Work out the finished part from the listing and answer in its coordinate system (mm). Face numbers are marked on the shaded views. A direction names the side the tool comes from. Round coordinates to 2 decimals unless told otherwise and drop trailing zeros. Write each loop counter-clockwise with the first axis right and the second up, starting at its lowest first coordinate (ties: lowest second). Pieces come first, ordered by that corner, then holes. Notation, with made-up numbers: (-22.5, 42) -> (-16.5, 42) arc R9 ccw to (-16.5, 54) -> close; hole circle Ø9 at (-3.5, 68). An arc over 180 degrees is marked (long way). One line per item, written item: value.
Solid Edge part; units mm, degrees
sketch "Sketch1" plane through (0, 0, 0) normal (1, 0, 0) x (0, 1, 0)
  line L0 (0, -1.4097) -> (0, 1.4097)
  arc A0 (0, 1.4097) -> (5.25, -1.4097) centre (0.36, -4.2176) cw
  line L1 (0, -1.4097) -> (5.25, -1.4097)
revolve "RevolvedProtrusion1" add sketch "Sketch1" angle 360 about axis through (0, 0, -14.7796) along (0, 0, 1)
sketch "Sketch2" plane through (0, 0, -1.4097) normal (0, 0, -1) x (0, 1, 0)
  circle A0 centre (0, 0) radius 3
extrude "Protrusion1" add sketch "Sketch2" along normal blind 20
sketch "Sketch3" plane through (0, 0, -21.4097) normal (0, 0, -1) x (1, 0, 0)
  circle A0 centre (0, 0) radius 2.9975
extrude "Cutout1" cut sketch "Sketch3" against normal blind 18.4125 flip side to cut
sketch "Sketch4" plane through (-0.6032, 0.3606, 2.8194) normal (0, 0, 1) x (1, 0, 0)
  line L0 (-0.5515, 1.6394) -> (1.7579, 1.6394)
  line L1 (2.9126, -0.3606) -> (1.7579, 1.6394)
  line L2 (1.7579, -2.3606) -> (2.9126, -0.3606)
  line L3 (-0.5515, -2.3606) -> (1.7579, -2.3606)
  line L4 (-1.7062, -0.3606) -> (-0.5515, -2.3606)
  line L5 (-0.5515, 1.6394) -> (-1.7062, -0.3606)
extrude "ExtrudedCutout_11" cut sketch "Sketch4" against normal blind 4.2291
fillet "Round_3" radius 0.5 1 edges at (3, 0, -1.4097)
properties part number "182126"
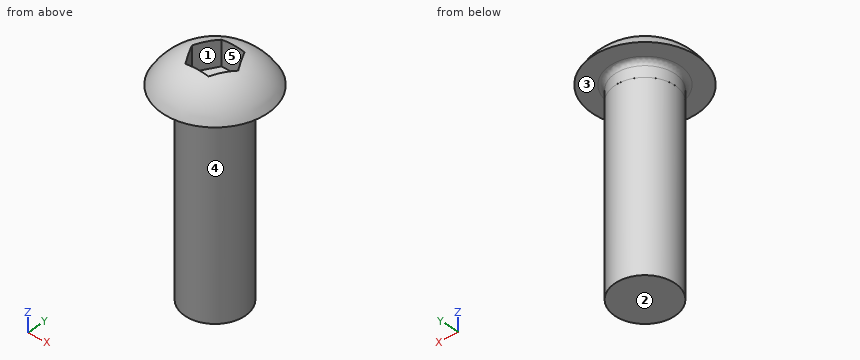
(1) Find section A-A on z = -11.5. Give the vertices of the cut face in (x, y) (1 decimal).
Reported:
outline: circle Ø6 at (0, 0)
(2) For a pull along Y with two mould halves and no side action, classify the marked faces 3, 4 and 5 as pulls with the +Y half, pulls with the -Y half, needs draft (parallel to the pull), parting line crosses it, or undercut.
Reported:
face 3: needs draft
face 4: parting line crosses it
face 5: undercut
(3) A tool of negligible diameter and unlimited length cuts with its end or side. For the marked faces 1 and 2, from which of +Z, -Z, +X, -X, +Y, -Y can it reach the whole face along a straight path? Write none if from no direction.
Reported:
face 1: +Z
face 2: -Z, +X, -X, +Y, -Y
(4) Flat-ended cylindrical pins translate along their axes: pin 1 Ø1.5 at (y, z) = (-0.5, -6.5) entering from -X; pin 2 Ø4 at (x, z) = (2, -8.5) entering from -Y; pin 3 Ø6 at (x, z) = (3.5, -3.5) entering from +Y. Find the tip coordinate at first contact, or state that the pin passes through.
Reported:
pin 1: stops at x = -3
pin 2: stops at y = -3
pin 3: stops at y = 5.07
(5) Consider probe 1 along Y at (x, z) = (-1.5, -0.75); probe 2 along X at (y, z) = (0, -10); probe 3 along Z at (x, y) = (-1.5, -3.25). Determine where each line is inside the solid, lowest interval first.
Reported:
probe 1: y = -4.57 to -1.4, 1.4 to 4.57
probe 2: x = -3 to 3
probe 3: z = -1.41 to 0.41
